from build123d import *

# Parameters (mm, degrees)
SKETCH1_W           = 18
SKETCH1_H           = 40.5
BOSS_EXTRUDE1_DEPTH = 4
SKETCH2_W           = 10
SKETCH2_H           = 4
BOSS_EXTRUDE2_DEPTH = 4
SKETCH3_W           = 10
SKETCH3_H           = 4
BOSS_EXTRUDE3_DEPTH = 6


with BuildPart() as part:
    # Sketch1 → Boss-Extrude1 (new body)
    with BuildSketch(Plane(origin=(0, 0, 0), x_dir=(1, 0, 0), z_dir=(0, 1, 0))):
        with Locations((9, -20.25)):
            Rectangle(SKETCH1_W, SKETCH1_H)
    extrude(amount=BOSS_EXTRUDE1_DEPTH)

    # Sketch2 → Boss-Extrude2 (add, through all)
    with BuildSketch(Plane(origin=(0, 0, 0), x_dir=(-1, 0, 0), z_dir=(0, -1, 0))):
        with Locations((-9, 2)):
            Rectangle(SKETCH2_W, SKETCH2_H)
        with Locations((-9, -42.5)):
            Rectangle(SKETCH2_W, SKETCH2_H)
    extrude(amount=-BOSS_EXTRUDE2_DEPTH)

    # Sketch3 → Boss-Extrude3 (add)
    with BuildSketch(Plane(origin=(18, 0, 0), x_dir=(0, 0, -1), z_dir=(1, 0, 0))):
        with Locations((-12.75, 2)):
            Rectangle(SKETCH3_W, SKETCH3_H)
        with Locations((-27.75, 2)):
            Rectangle(SKETCH3_W, SKETCH3_H)
    extrude(amount=BOSS_EXTRUDE3_DEPTH)


solid = part.part
The listing builds one solid part. Answer for the finished solid, in the listing's coordinates (mm). A direction names the side the tool comes from. Round coordinates to 2 decimals unless told otherwise and drop trailing zeros. Order: outer loops, then holes, each group sorted by start corner. A loop starts at its lowest first (then second) coordinate and runs counter-clockwise, first axis right, second up. Notation, with made-up numbers: M -24.75,51 L -12.75,51 A10 cw -12.75,56 Z; hole C 81,15 d3. An arc over 180 degrees is marked long. Answer in a Markdown table with one row per item. Add a question column.
1) The part is cut by section D-D on x = 15.75. Determine the outline of the cut face in (y, z), plus the area to 3 significant figures.
2) Flat-ended cylindrical pins translate along their axes: pin 1 Ø1.2 at (x, y) = (16.5, 1.5) entering from -Z; pin 2 Ø2 at (x, y) = (20.5, 1) entering from +Z; pin 3 Ø2 at (y, z) = (2, 37) entering from +X. Find the tip coordinate at first contact, or state that the pin passes through.
3) The part is cut by section C-C on z = 36.5. Determine the outline of the cut face in (x, y), plus the area to 3 significant figures.
4) Determine the mould class of faces 5 (the face through (21, 2, 17.75)), 6 (the face through (21, 2, 22.75)), 7 (the face through (9, 2, 44.5)), 8 (the face through (4, 2, 43)) for opening direction Z: pulls with the +Z half, pulls with the -Z half, needs draft (parallel to the pull), parting line crosses it, or undercut.
5) Which of the six approach directions +Z, -Z, +X, -X, +Y, -Y give full straight-line access (tool end or side, diameter ignored) to faces 1 (the face through (18, 2, 4)), 2 (the face through (2, 2, 40.5)), 3 (the face through (4, 2, -2)), 4 (the face through (14, 2, 43))?
6) Consider line 1 along Z through (x, y) = (19.25, 0.7); line 2 along X through (y, z) = (0.85, 35); line 3 along Z through (x, y) = (17.75, 3.05). Determine where each line is inside the solid, lowest interval first. Write a range as from..to.
7) The part is cut by section A-A on x = 18.75. Determine the outline of the cut face in (y, z).
8) The part is cut by section B-B on y = 0.45. Determine the outline of the cut face in (x, z).
Findings below:
| question | item | result |
|---|---|---|
| 1 | outline | M 0,0 L 4,0 L 4,40.5 L 0,40.5 Z |
| 1 | area | 162 mm² |
| 2 | pin 1 | stops at z = 0 |
| 2 | pin 2 | stops at z = 32.75 |
| 2 | pin 3 | stops at x = 18 |
| 3 | outline | M 0,0 L 18,0 L 18,4 L 0,4 Z |
| 3 | area | 72.0 mm² |
| 4 | face 5 | undercut |
| 4 | face 6 | undercut |
| 4 | face 7 | pulls with the +Z half |
| 4 | face 8 | needs draft |
| 5 | face 1 | -Z, +X, +Y, -Y |
| 5 | face 2 | +Z, -X, +Y, -Y |
| 5 | face 3 | -Z, -X, +Y, -Y |
| 5 | face 4 | +Z, +X, +Y, -Y |
| 6 | line 1 | z = 7.75..17.75, 22.75..32.75 |
| 6 | line 2 | x = 0..18 |
| 6 | line 3 | z = 0..40.5 |
| 7 | outline | M 0,7.75 L 4,7.75 L 4,17.75 L 0,17.75 Z; M 0,22.75 L 4,22.75 L 4,32.75 L 0,32.75 Z |
| 8 | outline | M 0,0 L 4,0 L 4,-4 L 14,-4 L 14,0 L 18,0 L 18,7.75 L 24,7.75 L 24,17.75 L 18,17.75 L 18,22.75 L 24,22.75 L 24,32.75 L 18,32.75 L 18,40.5 L 14,40.5 L 14,44.5 L 4,44.5 L 4,40.5 L 0,40.5 Z |
